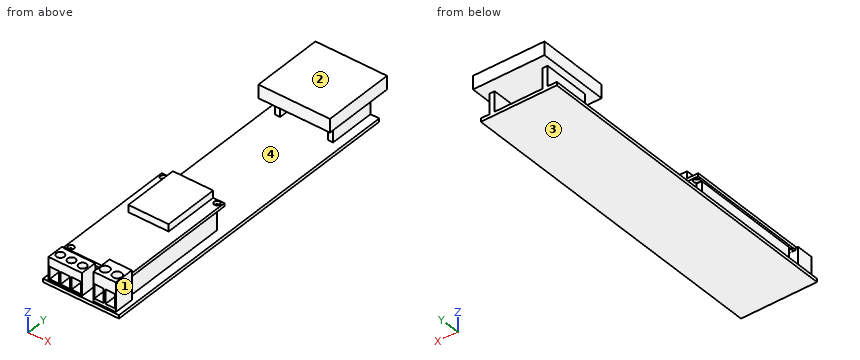
from build123d import *

# Parameters (mm, degrees)
SKICA1_W                    = 34
SKICA1_H                    = 146
PCB_DEPTH                   = 1.5
SKICA2_W                    = 10
SKICA2_H                    = 9
T_LO_DEPTH                  = 13
SKICA3_W                    = 4.2
SKICA3_H                    = 6.4
D_RA_NA_DR_TKY_DEPTH        = 6
SKICA4_R                    = 2
D_RY_NA_ROUBKY_DEPTH        = 5.2
SKICA5_W                    = 15
SKICA5_H                    = 7.6
T_LO_LOGIKY_KONEKTORU_DEPTH = 10
SKICA6_W                    = 4.2
SKICA6_H                    = 5.5
D_RY_NA_DR_TKY_DEPTH        = 6
SKICA7_R                    = 1.75
D_RY_NA_KOUBKY_DEPTH        = 4
SKICA8_W                    = 2.3
SKICA8_H                    = 49
LI_TY_DEPTH                 = 9
SKICA9_W                    = 28
SKICA9_H                    = 55
SKICA9_R                    = 1.3
PCB_ESP32_BOARD_DEPTH       = 1.4
SKICA10_W                   = 18
SKICA10_H                   = 25
CHIP_ESP32_DEPTH            = 3.2
SKICA11_W                   = 2.3
SKICA11_H                   = 21
LISTY_DEPTH                 = 9
SKICA12_W                   = 32
SKICA12_H                   = 32
F_8X8_LED_MATICE_DEPTH      = 6


with BuildPart() as part:
    # Skica1 → PCB (new body)
    with BuildSketch(Plane.XY):
        with Locations((17, 73)):
            Rectangle(SKICA1_W, SKICA1_H)
    extrude(amount=PCB_DEPTH)

    # Skica2 → tělo (add)
    with BuildSketch(Plane.XY.offset(1.5)):
        with Locations((27, 5.2)):
            Rectangle(SKICA2_W, SKICA2_H)
    extrude(amount=T_LO_DEPTH)

    # Skica3 → díra na drátky (cut)
    with BuildSketch(Plane.XZ.offset(-0.7)):
        with Locations((24.5, 6.1)):
            Rectangle(SKICA3_W, SKICA3_H)
        with Locations((29.5, 6.1)):
            Rectangle(SKICA3_W, SKICA3_H)
    extrude(amount=-D_RA_NA_DR_TKY_DEPTH, mode=Mode.SUBTRACT)

    # Skica4 → díry na šroubky (cut)
    with BuildSketch(Plane.XY.offset(14.5)):
        with Locations((29.7, 4.4)):
            Circle(SKICA4_R)
        with Locations((24.3, 4.4)):
            Circle(SKICA4_R)
    extrude(amount=-D_RY_NA_ROUBKY_DEPTH, mode=Mode.SUBTRACT)

    # Skica5 → tělo logiky konektoru (add)
    with BuildSketch(Plane.XY.offset(1.5)):
        with Locations((9.4, 4.5)):
            Rectangle(SKICA5_W, SKICA5_H)
    extrude(amount=T_LO_LOGIKY_KONEKTORU_DEPTH)

    # Skica6 → díry na drátky (cut)
    with BuildSketch(Plane.XZ.offset(-0.7)):
        with Locations((4.5, 4.75)):
            Rectangle(SKICA6_W, SKICA6_H)
        with Locations((9.4, 4.75)):
            Rectangle(SKICA6_W, SKICA6_H)
        with Locations((14.3, 4.75)):
            Rectangle(SKICA6_W, SKICA6_H)
    extrude(amount=-D_RY_NA_DR_TKY_DEPTH, mode=Mode.SUBTRACT)

    # Skica7 → díry na škoubky (cut)
    with BuildSketch(Plane.XY.offset(11.5)):
        with Locations((4.4, 4.2)):
            Circle(SKICA7_R)
        with Locations((9.4, 4.2)):
            Circle(SKICA7_R)
        with Locations((14.4, 4.2)):
            Circle(SKICA7_R)
    extrude(amount=-D_RY_NA_KOUBKY_DEPTH, mode=Mode.SUBTRACT)

    # Skica8 → lišty (add)
    with BuildSketch(Plane.XY.offset(1.5)):
        with Locations((4.85, 35.5)):
            Rectangle(SKICA8_W, SKICA8_H)
        with Locations((28.95, 35.5)):
            Rectangle(SKICA8_W, SKICA8_H)
    extrude(amount=LI_TY_DEPTH)



with BuildPart() as body_2:
    # Skica9 → PCB ESP32 board (new body)
    with BuildSketch(Plane.XY.offset(10.5)):
        with Locations((16.9, 35.5)):
            Rectangle(SKICA9_W, SKICA9_H)
        with Locations((28.9, 61.4)):
            Circle(SKICA9_R, mode=Mode.SUBTRACT)
        with Locations((4.9, 61.4)):
            Circle(SKICA9_R, mode=Mode.SUBTRACT)
        with Locations((4.9, 9.6)):
            Circle(SKICA9_R, mode=Mode.SUBTRACT)
        with Locations((28.9, 9.6)):
            Circle(SKICA9_R, mode=Mode.SUBTRACT)
    extrude(amount=PCB_ESP32_BOARD_DEPTH)


with BuildPart() as part_1:
    add(part.part)

    add(body_2.part)  # chip ESP32 merges body 2
    # Skica10 → chip ESP32 (add)
    with BuildSketch(Plane.XY.offset(11.9)):
        with Locations((16.9, 50.5)):
            Rectangle(SKICA10_W, SKICA10_H)
    extrude(amount=CHIP_ESP32_DEPTH)

    # Skica11 → listy (add)
    with BuildSketch(Plane.XY.offset(1.5)):
        with Locations((28.95, 135.5)):
            Rectangle(SKICA11_W, SKICA11_H)
        with Locations((5.25, 135.5)):
            Rectangle(SKICA11_W, SKICA11_H)
    extrude(amount=LISTY_DEPTH)

    # Skica12 → 8x8 LED matice (add)
    with BuildSketch(Plane.XY.offset(10.5)):
        with Locations((17.1, 135.5)):
            Rectangle(SKICA12_W, SKICA12_H)
    extrude(amount=F_8X8_LED_MATICE_DEPTH)


solid = part_1.part
Geometry check sheet. Reference: the model listing, model coordinates, mm. Face numbers are marked on the shaded views. Round coordinates to 2 decimals unless told otherwise and drop trailing zeros. Write each loop counter-clockwise with the first axis right and the second up, starting at its lowest first coordinate (ties: lowest second). Pieces come first, ordered by that corner, then holes. Notation, with made-up numbers: (-37.5, -25.75) - (1.5, -25.75) arc R28 ccw to (1.5, 0.25) - close; hole circle Ø9 at (-5, 41.5). An arc over 180 degrees is marked (long way). One line per item, written item: value.
1. Depth check by flat-ended pin: pin 1 Ø3 at (x, y) = (14.4, 4.2) entering from +Z; pin 2 Ø2 at (x, z) = (26, 8) entering from -Y; pin 3 Ø12 at (x, y) = (9, 44) entering from +Z; pin 4 Ø4.5 at (x, z) = (9, 3.5) entering from -Y. Enter the tip coordinate at first touch or a pass-through.
The answers:
pin 1: stops at z = 2
pin 2: stops at y = 0.7
pin 3: stops at z = 15.1
pin 4: stops at y = 0
2. Cross-section at B-B on y = 32.5. Record the boundary of the cut face in (x, z).
The answers:
outline: (0, 0) - (34, 0) - (34, 1.5) - (30.1, 1.5) - (30.1, 10.5) - (30.9, 10.5) - (30.9, 11.9) - (2.9, 11.9) - (2.9, 10.5) - (3.7, 10.5) - (3.7, 1.5) - (0, 1.5) - close; hole (6, 1.5) - (27.8, 1.5) - (27.8, 10.5) - (6, 10.5) - close
3. Cross-section at A-A on x = 9.4. Record the boundary of the cut face in (y, z).
The answers:
outline: (0, 0) - (146, 0) - (146, 1.5) - (8.3, 1.5) - (8.3, 10.5) - (63, 10.5) - (63, 15.1) - (38, 15.1) - (38, 11.9) - (8, 11.9) - (8, 11.5) - (5.95, 11.5) - (5.95, 7.5) - (6.7, 7.5) - (6.7, 2) - (0.7, 2) - (0.7, 1.5) - (0, 1.5) - close; (0.7, 7.5) - (2.45, 7.5) - (2.45, 11.5) - (0.7, 11.5) - close; (119.5, 10.5) - (151.5, 10.5) - (151.5, 16.5) - (119.5, 16.5) - close
4. Scan lines: L1, parallel to Y at x = 4.4, z = 9.7; L2, parallel to Y at x = 28, z = 2; L3, parallel to X at y = 4.4, z = 13.2. Record each from-to range of solid material in increasing order.
The answers:
L1: y = 0.7 to 2.45, 5.95 to 8.3, 11 to 60, 125 to 146
L2: y = 0.7 to 9.7, 11 to 60, 125 to 146
L3: x = 22 to 22.3, 26.3 to 27.7, 31.7 to 32
5. Cross-section at D-D on x = 24.3. Record the boundary of the cut face in (y, z).
The answers:
outline: (0, 0) - (146, 0) - (146, 1.5) - (9.7, 1.5) - (9.7, 10.5) - (63, 10.5) - (63, 15.1) - (38, 15.1) - (38, 11.9) - (9.7, 11.9) - (9.7, 14.5) - (6.4, 14.5) - (6.4, 9.3) - (6.7, 9.3) - (6.7, 2.9) - (0.7, 2.9) - (0.7, 1.5) - (0, 1.5) - close; (0.7, 9.3) - (2.4, 9.3) - (2.4, 14.5) - (0.7, 14.5) - close; (119.5, 10.5) - (151.5, 10.5) - (151.5, 16.5) - (119.5, 16.5) - close
6. Cross-section at C-C on z = 5.5. Give the number of separate pieces and of enclosed holes in the cut face, and give its area (3 significant figures).
The answers:
separate pieces: 6
enclosed holes: 0
area: 400 mm^2
7. Mould release check, pull along Z, two halves, no side actions. Record for the marked faces 1, 2, 3 and 4: released by +Z, released by -Z, zero draft, split by the parting line, or undercut.
The answers:
face 1: zero draft
face 2: released by +Z
face 3: released by -Z
face 4: undercut
